For this review, use the dimensioned drawing (mm, ordinates from the lowest corner) and the shaded views. A direction names the side the tool comes from. Give positions to 0.01 mm unless a question says otherwise; leave off trailing zeros. Write each loop counter-clockwise with the first axis right and the second up, starting at its lowest first coordinate (ties: lowest second). Pieces come first, ordered by that corner, then holes. Notation, with made-up numbers: M 78,-13 L 122,-13 A24 cw 122,7 Z; hole C -14,78.25 d8. An arc over 180 degrees is marked long. Use a Markdown table: item, result. Add a question column.
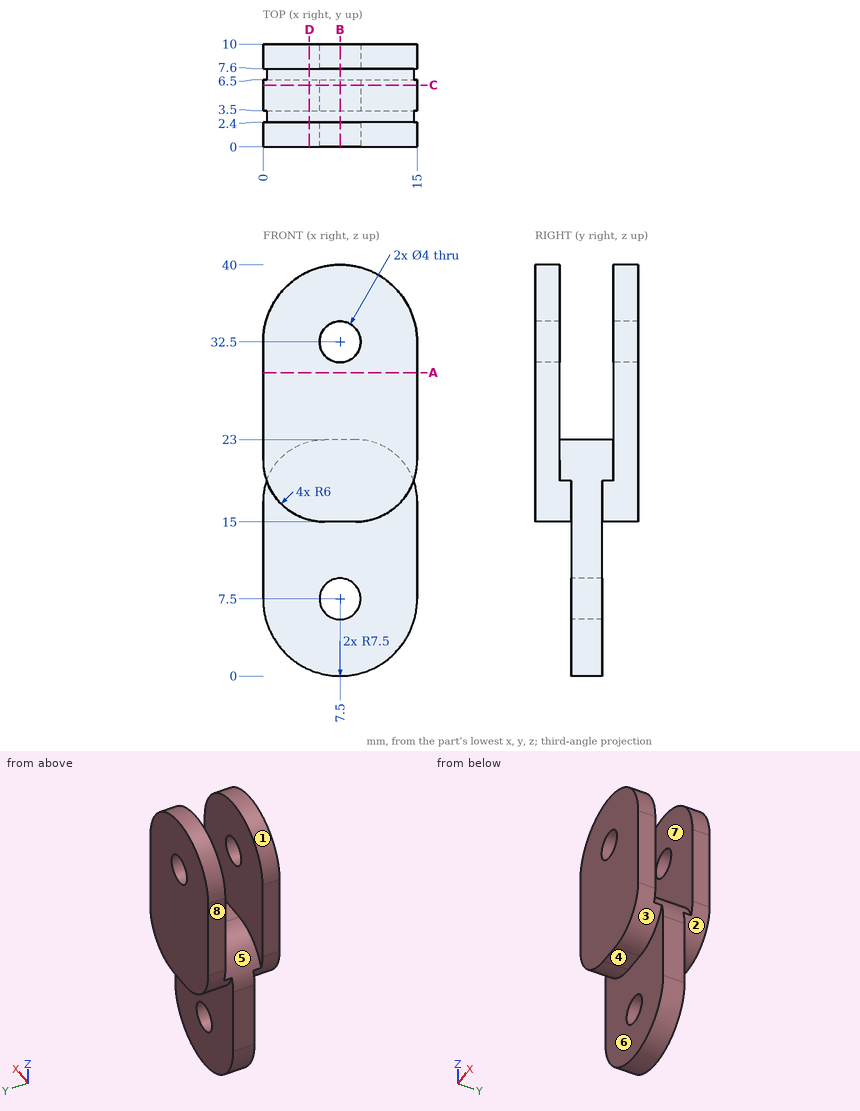
(1) Add section A-A on z = 29.5. Give the boundary of the cut face in (x, y), then the cut area to 3 significant figures.
(2) Add section C-C on y = 6. Give the boundary of the cut face in (x, z).
(3) Add section D-D on x = 4.5. Give the boundary of the cut face in (y, z), then the cut area to 3 significant figures.
(4) Add section B-B on x = 7.5. Give the boundary of the cut face in (y, z), then the cut area to 3 significant figures.
(5) The part is to be moulded in two halves that separate along Y. For the marked faces 5, 6, 7 and 8, say which applies: released by +Y, released by -Y, zero draft, split by the parting line, or undercut.
(6) Wall thickness on L1, parallel to Y at x = 9.25, z = 28.5; L2, parallel to Z at x = 7.5, y = 1.5; L3, parallel to Z at x = 7.5, y = 5.15: over which ranges is each line inside the solid? List them lowest first.
(7) For pin 1 (3 mm diameter, centred on x = 7.5, z = 32.5, fed in from -Y); pin 2 (5 mm diameter, centred on x = 10.5, y = 8, fed in from -Z); pin 3 (2 mm diameter, centred on x = 1.5, y = 2, fed in from +Z); pin 4 (0.9 mm diameter, centred on x = 7.5, y = 5, fed in from +Z), all flat-tipped, find the tip position at first contact; note any pin that passes through.
(8) Machinability: for the marked faces 1, 2, 3 and 4, which of the approach directions +Z, -Z, +X, -X, +Y, -Y give a long, thin tool a straight path to every point of the face, cutting with its end or side? Answer none if there is none.
From the geometry:
| question | item | result |
|---|---|---|
| 1 | outline | M 0,0 L 15,0 L 15,2.4 L 0,2.4 Z; M 0,7.6 L 15,7.6 L 15,10 L 0,10 Z |
| 1 | area | 72.0 mm^2 |
| 2 | outline | M 0,7.5 A7.5 ccw 15,7.5 L 15,17 A6 ccw 9,23 L 6,23 A6 ccw 0,17 Z; hole C 7.5,7.5 d4 |
| 3 | outline | M 0,15.19 L 3.5,15.19 L 3.5,0.63 L 6.5,0.63 L 6.5,15.19 L 10,15.19 L 10,39.37 L 7.6,39.37 L 7.6,22.81 L 2.4,22.81 L 2.4,39.37 L 0,39.37 Z |
| 3 | area | 199 mm^2 |
| 4 | outline | M 0,15 L 3.5,15 L 3.5,9.5 L 6.5,9.5 L 6.5,15 L 10,15 L 10,30.5 L 7.6,30.5 L 7.6,23 L 2.4,23 L 2.4,30.5 L 0,30.5 Z; M 0,34.5 L 2.4,34.5 L 2.4,40 L 0,40 Z; M 3.5,0 L 6.5,0 L 6.5,5.5 L 3.5,5.5 Z; M 7.6,34.5 L 10,34.5 L 10,40 L 7.6,40 Z |
| 4 | area | 175 mm^2 |
| 5 | face 5 | undercut |
| 5 | face 6 | released by -Y |
| 5 | face 7 | undercut |
| 5 | face 8 | zero draft |
| 6 | L1 | y = 0 to 2.4, 7.6 to 10 |
| 6 | L2 | z = 15 to 30.5, 34.5 to 40 |
| 6 | L3 | z = 0 to 5.5, 9.5 to 23 |
| 7 | pin 1 | passes through |
| 7 | pin 2 | stops at z = 0.07 |
| 7 | pin 3 | stops at z = 38.09 |
| 7 | pin 4 | stops at z = 23 |
| 8 | face 1 | +Z, +Y, -Y |
| 8 | face 2 | -Z, +X, +Y |
| 8 | face 3 | -Z, +X, -Y |
| 8 | face 4 | -Z, +X, -X, -Y |
